Part model, mm, in its own coordinate system. Face numbers are marked on the shaded views. A direction names the side the tool comes from. Round coordinates to 2 decimals unless told otherwise and drop trailing zeros. Write each loop counter-clockwise with the first axis right and the second up, starting at its lowest first coordinate (ties: lowest second). Pieces come first, ordered by that corner, then holes.
1) Saw through at B-B on x = 0. Write the cut outline in (y, z).
2) Saw through at A-A on y = 23.5. Write the cut outline in (x, z).
3) Which spindle directions (+Z, -Z, +X, -X, +Y, -Y) get a long thin tool onto all of the face, cutting with end or side? Do the marked faces 1, 2, 3, 4 and 5. Say none if no direction does.
4) Flat gauge pins, fed straight in: pin 1 (8 mm diameter, centred on x = 4.5, z = 6.5, fed in from -Y); pin 2 (4 mm diameter, centred on x = 0, y = 26.5, fed in from -Z); pin 3 (4 mm diameter, centred on x = 0.5, y = 17.5, fed in from -Z); pin 4 (2 mm diameter, centred on x = -8.5, y = 21, fed in from -Z). Where does each tip first touch, or does it go through?
5) Drill centre lines: L1, parallel to X at y = 12.25, z = 0; L2, parallel to X at y = 20.5, z = 0; L3, parallel to Y at x = 7.5, z = -9. Where is each one in solid material? Low to high.
6) Saw through at D-D on x = -9. Write the cut outline in (y, z).
7) Saw through at C-C on z = 11.5. Write the cut outline in (x, y).
8) Pull direction Z, two halves, no side cores. Call the marked faces 6, 7 and 8: +Z half, -Z half, draft (parallel to the pull), parting line (faces both ways), or undercut.
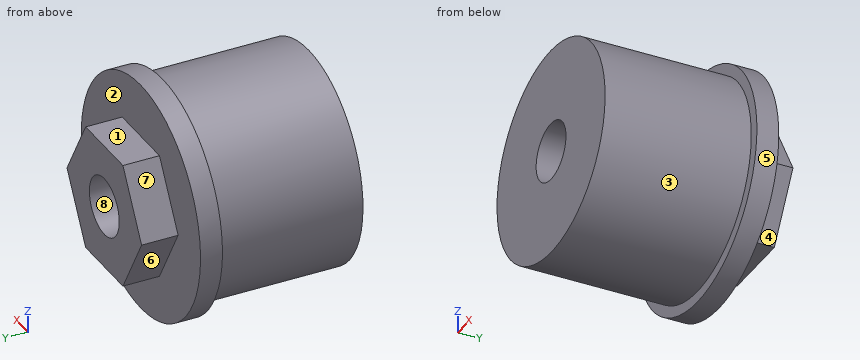
```python
from build123d import *

# Parameters (mm, degrees)
SKETCH1_R           = 14.5
BOSS_EXTRUDE1_DEPTH = 20
SKETCH2_R           = 16
BOSS_EXTRUDE2_DEPTH = 3
BOSS_EXTRUDE3_DEPTH = 5
SKETCH4_R           = 4
CUT_EXTRUDE1_DEPTH  = 30


with BuildPart() as part:
    # Sketch1 → Boss-Extrude1 (new body)
    with BuildSketch(Plane(origin=(0, 0, 0), x_dir=(1, 0, 0), z_dir=(0, 1, 0))):
        with Locations(Location((0, 0, 0), (0, 0, 270))):
            Circle(SKETCH1_R)
    extrude(amount=BOSS_EXTRUDE1_DEPTH)

    # Sketch2 → Boss-Extrude2 (add)
    with BuildSketch(Plane(origin=(0, 20, 0), x_dir=(1, 0, 0), z_dir=(0, 1, 0))):
        with Locations(Location((0, 0, 0), (0, 0, 270))):
            Circle(SKETCH2_R)
    extrude(amount=BOSS_EXTRUDE2_DEPTH)

    # Sketch3 → Boss-Extrude3 (add)
    with BuildSketch(Plane(origin=(0, 23, 0), x_dir=(1, 0, 0), z_dir=(0, 1, 0))):
        Polygon((10, 0), (5, 8.660254038), (-5, 8.660254038), (-10, 0), (-5, -8.660254038), (5, -8.660254038), align=None)
    extrude(amount=BOSS_EXTRUDE3_DEPTH)

    # Sketch4 → Cut-Extrude1 (cut)
    with BuildSketch(Plane(origin=(0, 28, 0), x_dir=(1, 0, 0), z_dir=(0, 1, 0))):
        with Locations(Location((0, 0, 0), (0, 0, 270))):
            Circle(SKETCH4_R)
    extrude(amount=-CUT_EXTRUDE1_DEPTH, mode=Mode.SUBTRACT)


solid = part.part
```
Completed:
1. outline: (0, -14.5) - (20, -14.5) - (20, -16) - (23, -16) - (23, -8.66) - (28, -8.66) - (28, -4) - (0, -4) - close; (0, 4) - (28, 4) - (28, 8.66) - (23, 8.66) - (23, 16) - (20, 16) - (20, 14.5) - (0, 14.5) - close
2. outline: (-10, 0) - (-5, -8.66) - (5, -8.66) - (10, 0) - (5, 8.66) - (-5, 8.66) - close; hole circle Ø8 at (0, 0)
3. face 1: +Z, +X, -X, +Y
3. face 2: +Y
3. face 3: -Y
3. face 4: -Z, +X, +Y
3. face 5: +Y, -Y
4. pin 1: stops at y = 0
4. pin 2: stops at z = -8.66
4. pin 3: stops at z = -14.5
4. pin 4: stops at z = -14.13
5. L1: x = -14.5 to -4, 4 to 14.5
5. L2: x = -16 to -4, 4 to 16
5. L3: y = 0 to 23
6. outline: (0, -11.37) - (20, -11.37) - (20, -13.23) - (23, -13.23) - (23, -1.73) - (28, -1.73) - (28, 1.73) - (23, 1.73) - (23, 13.23) - (20, 13.23) - (20, 11.37) - (0, 11.37) - close
7. outline: (-11.12, 20) - (-8.83, 20) - (-8.83, 0) - (8.83, 0) - (8.83, 20) - (11.12, 20) - (11.12, 23) - (-11.12, 23) - close
8. face 6: -Z half
8. face 7: +Z half
8. face 8: undercut
